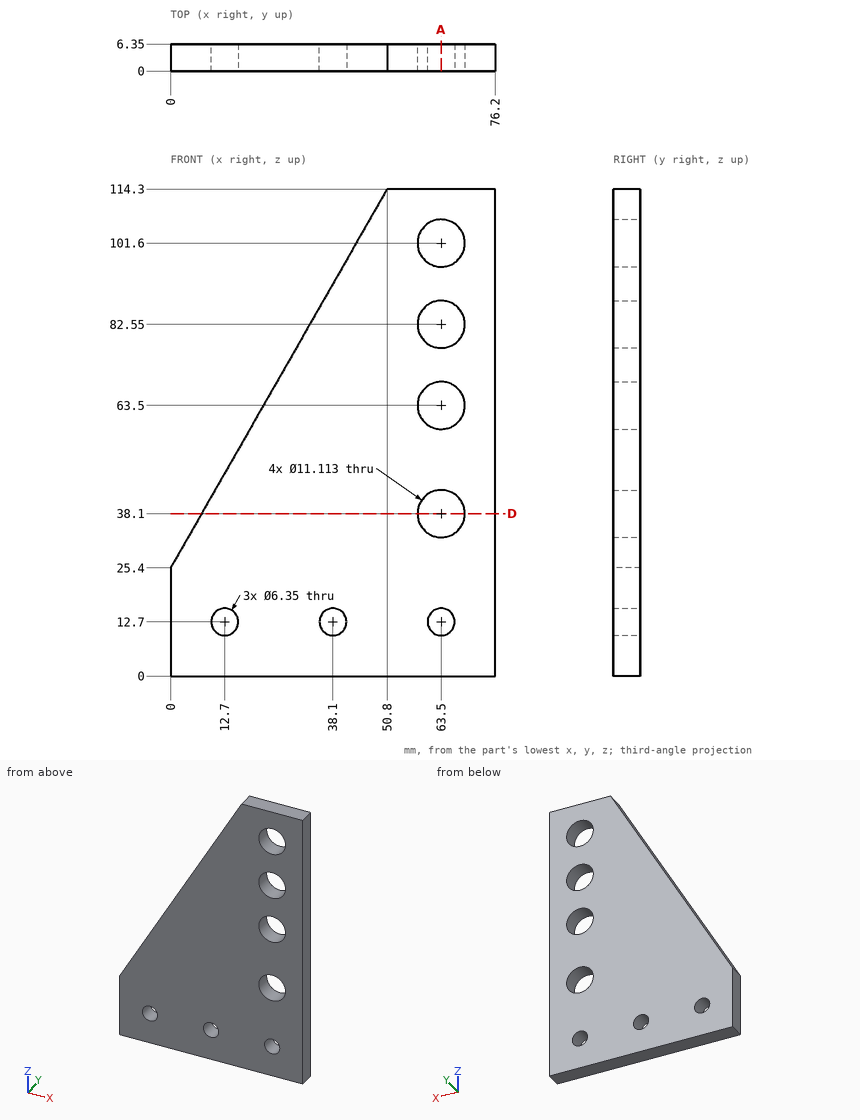
Check sheet for the drawn part. Datum: minimum x, y, z corner. Units: mm. Round coordinates to 2 decimals unless told otherwise and drop trailing zeros. Loops run counter-clockwise (first coordinate to the right, second up) from the corner with the lowest first, then second, coordinate; pieces in that order, holes last. Notation, with made-up numbers: (26, 46.25) - (65, 46.25) arc R12 ccw to (65, 68.25) - close; hole circle Ø8 at (12, 54.5). An arc over 180 degrees is marked (long way). Write item = value, one per line. Start each with the question number.
1. Section check D-D on z = 38.1. Enter the section's corners in (x, y).
2. Thickness scan on line 1 (Z direction, x = 63.5, y = 1.5) (1 decimal); line 2 (X direction, y = 5.75, z = 12.5); line 3 (Z direction, x = 65, y = 1.25). Record the ranges inside material, lowest first.
3. Depth check by flat-ended pin: pin 1 (14.5 mm diameter, centred on x = 63.5, z = 63.5, fed in from +Y); pin 2 (1.5 mm diameter, centred on y = 3.5, z = 74, fed in from -X). Enter the tip coordinate at first touch or a pass-through.
4. Section check A-A on x = 63.5. Give the number of separate pieces and of enclosed holes in the cut face, then the cut area to 3 significant figures.
Working result:
q1.outline = (7.26, 0) - (57.94, 0) - (57.94, 6.35) - (7.26, 6.35) - close; (69.06, 0) - (76.2, 0) - (76.2, 6.35) - (69.06, 6.35) - close
q2.line_1 = 0 to 9.5, 15.9 to 32.5, 43.7 to 57.9, 69.1 to 77, 88.1 to 96, 107.2 to 114.3
q2.line_2 = 0 to 9.53, 15.87 to 34.93, 41.27 to 60.33, 66.67 to 76.2
q2.line_3 = 0 to 9.9, 15.5 to 32.75, 43.45 to 58.15, 68.85 to 77.2, 87.9 to 96.25, 106.95 to 114.3
q3.pin_1 = 6.35
q3.pin_2 = 27.34
q4.separate_pieces = 6
q4.enclosed_holes = 0
q4.area = 403 mm^2
